Could you check a few things on this model? Use its own coordinates, in mm. A direction names the side the tool comes from. Round coordinates to 2 decimals unless told otherwise and drop trailing zeros. Loops run counter-clockwise (first coordinate to the right, second up) from the corner with the lowest first, then second, coordinate; pieces in that order, holes last. Notation, with made-up numbers: (11, 34) - (27, 34) arc R21 ccw to (27, 53) - close; hole circle Ø10 at (65.25, 54). An arc over 180 degrees is marked (long way). Put each result on its own line as item: value. Start each with the question number.
from build123d import *

# Parameters (mm, degrees)
SKETCH_1_R               = 87.5
EXTRUDE_1_DEPTH          = 150
EXTRUDE_2_DEPTH          = 150
PATTERN_CIRCULAR_1_COUNT = 20
CUT_EXTRUDE_1_DEPTH      = 217.10182785
FILLET_1_R               = 3


with BuildPart() as part:
    # 草图1 → 拉伸1 (new body)
    with BuildSketch(Plane.XY):
        Circle(SKETCH_1_R)
    extrude(amount=EXTRUDE_1_DEPTH)

    # 草图2 → 拉伸2 (add)
    with BuildSketch(Plane.XY):
        with BuildLine():
            ThreePointArc((10, 86.926693254), (0, 87.5), (-10, 86.926693254))
            ThreePointArc((-10, 86.926693254), (-8.101258535, 98.817083904), (-3.5, 109.944304082))
            ThreePointArc((-3.5, 109.944304082), (0, 110), (3.5, 109.944304082))
            ThreePointArc((3.5, 109.944304082), (8.101258535, 98.817083904), (10, 86.926693254))
        make_face()
    extrude_2 = extrude(amount=EXTRUDE_2_DEPTH)

    # 阵列(圆周)1: 拉伸2 ×20 about axis
    pattern_circular_1_axis = Axis((0, 0, 0), (0, 0, 1))
    for i in range(1, PATTERN_CIRCULAR_1_COUNT):
        add(extrude_2.rotate(pattern_circular_1_axis, i * 360 / PATTERN_CIRCULAR_1_COUNT))

    # 草图3 → 切除-拉伸1 (cut, through all)
    with BuildSketch(Plane.XY):
        with BuildLine():
            Line((57.827329179, 16), (67, 16))
            Line((67, 16), (67, -16))
            Line((67, -16), (57.827329179, -16))
            ThreePointArc((57.827329179, -16), (-60, 0), (57.827329179, 16))
        make_face()
    extrude(amount=CUT_EXTRUDE_1_DEPTH, mode=Mode.SUBTRACT)

    # 圆角1
    fillet_1_edges = [part.edges().sort_by_distance(p)[0] for p in [
        (-60, 0, 0),
        (-60, 0, 150),
    ]]
    fillet(fillet_1_edges, radius=FILLET_1_R)


solid = part.part
Item 1: Will these pins go through, and if not, where does the flat tip stop? P1, Ø10, axis at y = -33, z = 121, coming from the -X side; P2, Ø4.5, axis at x = 62.5, z = 50, coming from the -Y side; P3, Ø12, axis at y = -72, z = 80.5, coming from the +X side.
Item 2: Suppose I cut it at A-A, the plane y = 0. List the corners of the cut face in (x, z) for me, then the cut area to 3 significant figures.
Item 3: Thinking about a two-plate mould opening in X: for faces 1 (the face through (-8.15, 98.65, 73.95)), 2 (the face through (98.98, -8.055, 73.95)), 3 (the face through (-98.98, 8.055, 73.95)), which applies, released by +X, released by -X, zero draft, split by the parting line, or undercut?
Item 4: On a 3-axis mill with a long thin cutter (end or side, diameter ignored), from which of +Z, -Z, +X, -X, +Y, -Y can I reach the whole of each face in a straight line? I mean faces 4 (the face through (8.055, 98.98, 73.95)), 5 (the face through (91.646, -38.247, 73.95)), 6 (the face through (96.624, 22.926, 73.95)), 7 (the face through (22.926, -96.624, 73.95)). Say none if no direction works.
Item 5: I need wall thicknesses on line 1 (X direction, y = 0, z = 95); line 2 (Y direction, x = 0, z = 33); line 3 (Y direction, x = 98.5, z = 105.5). Which ranges of each line are inside material? Lowest first, please. Write a range as from..to.
Numbers:
1. P1: x = -105.64
1. P2: y = -91
1. P3: x = 88
2. outline: (-110, 0) - (-63, 0) arc R3 ccw to (-60, 3) - (-60, 147) arc R3 ccw to (-63, 150) - (-110, 150) - close; (67, 0) - (110, 0) - (110, 150) - (67, 150) - close
2. area: 13,900 mm^2
3. face 1: undercut
3. face 2: released by +X
3. face 3: released by -X
4. face 4: +Z, -Z, +Y
4. face 5: +Z, -Z
4. face 6: +Z, -Z, +X
4. face 7: +Z, -Z, -Y
5. line 1: -110..-60, 67..110
5. line 2: -110..-60, 60..110
5. line 3: -38.04..-24.25, -8.19..8.19, 24.25..38.04
